The model under review builds one solid part; all positions refer to its coordinate system, in mm. A direction names the side the tool comes from. Coordinates: 2 decimals unless noted, no trailing zeros. Write each loop counter-clockwise with the first axis right and the second up, starting at its lowest first coordinate (ties: lowest second). Pieces come first, ordered by that corner, then holes.
1) Add section A-A, the plane y = 0. Give the number of separate pieces and of enclosed holes in the cut face, then the cut area to 3 significant figures.
2) For line 1 (Y direction, x = 1.25, z = -1.5); line 2 (Y direction, x = 2.75, z = 0); line 3 (Y direction, x = 4.5, z = 0), list the stretches that pass through material, from the lowest coordinate up.
3) Mouldability with a two-part tool opening along Z and no side actions: class faces 4 (the flat face through (0, 3, -3)), 5 (the conical face through (3.08, -0.63, -14.27)), 6 (the cylindrical face through (3.219, 3.514, -7.457)) as released by +Z, released by -Z, zero draft, split by the parting line, or undercut.
4) Add section B-B, the plane x = 2.75. State the section outline as (y, z) points (1 decimal), then the cut area to 3 significant figures.
5) Machinability: for faces 1 (the cylindrical face through (3.219, 0.445, 6.833)), 2 (the flat face through (6.35, 3, 3)), 3 (the conical face through (3.294, 12.703, 6.607)), which of the approach directions +Z, -Z, +X, -X, +Y, -Y give a long, thin tool a straight path to every point of the face, cutting with its end or side? Answer none if there is none.
6) For P1, Ø1.5, axis at x = 2, z = 12, coming from the -Y side; P2, Ø2, axis at x = 1, y = 10, coming from the -Z side; P3, Ø1.5, axis at x = 3, z = -9, coming from the -Y side, all flat-tipped, find the tip position at first contact; note any pin that passes through.
from build123d import *

# Parameters (mm, degrees)
CUT_EXTRUDE1_DEPTH      = 25.4561342
CUT_EXTRUDE1_DEPTH_BACK = 25.4561342


with BuildPart() as part:
    # Sketch1 → Revolve1 (revolve)
    with BuildSketch(Plane.XY, mode=Mode.PRIVATE) as revolve1_sk:
        Polygon((1.27, 16.7), (3.175, 14.16), (5.08, 16.7), (6.35, 16.7), (6.35, 4), (0, 4), (0, 16.7), align=None)
    revolve(revolve1_sk.sketch.rotate(Axis((0, 0, 0), (1, 0, 0)), 90), axis=Axis((0, 0, 0), (1, 0, 0)))

    # Sketch2 → Cut-Extrude1 (cut, two sides: drawn at the far end of the back side and taken through both)
    with BuildSketch(Plane.ZY.offset(-CUT_EXTRUDE1_DEPTH_BACK)):
        with BuildLine():
            ThreePointArc((-5.174909182, -4.484253782), (-6.96638667, -4.356158459), (-7.094481993, -6.147635947))
            ThreePointArc((-7.094481993, -6.147635947), (-4.201848282, -8.394615744), (-0.66952126, -9.363591392))
            ThreePointArc((-0.66952126, -9.363591392), (0.687821691, -8.187402584), (-0.488367117, -6.830059633))
            ThreePointArc((-0.488367117, -6.830059633), (-3.064943047, -6.123262296), (-5.174909182, -4.484253782))
        make_face()
        with BuildLine():
            ThreePointArc((-1.296023102, 6.723729704), (-0.289350555, 8.211147057), (-1.776767907, 9.217819605))
            ThreePointArc((-1.776767907, 9.217819605), (-5.169026349, 7.836215226), (-7.774347387, 5.261618115))
            ThreePointArc((-7.774347387, 5.261618115), (-7.434409475, 3.498030233), (-5.670821594, 3.837968145))
            ThreePointArc((-5.670821594, 3.837968145), (-3.77042918, 5.715949687), (-1.296023102, 6.723729704))
        make_face()
        with BuildLine():
            ThreePointArc((6.470932282, -2.239475923), (7.255737222, -3.854988599), (8.871249898, -3.070183659))
            ThreePointArc((8.871249898, -3.070183659), (9.370874629, 0.558400517), (8.443868645, 4.101973277))
            ThreePointArc((8.443868645, 4.101973277), (6.746587782, 4.68937235), (6.159188708, 2.992091487))
            ThreePointArc((6.159188708, 2.992091487), (6.835372224, 0.407312608), (6.470932282, -2.239475923))
        make_face()
    extrude(amount=CUT_EXTRUDE1_DEPTH + CUT_EXTRUDE1_DEPTH_BACK, mode=Mode.SUBTRACT)


solid = part.part
Geometry results:
1. separate pieces: 3
1. enclosed holes: 0
1. area: 135 mm2
2. line 1: y = -16.63 to -9.27, -6.68 to -3.71, 3.71 to 6.68, 9.24 to 16.63
2. line 2: y = -14.73 to -9.23, -6.97 to -4, 4 to 14.73
2. line 3: y = -15.93 to -9.23, -6.97 to -4, 4 to 15.93
3. face 4: zero draft
3. face 5: split by the parting line
3. face 6: undercut
4. outline: circle Ø29.5 at (0, 0); hole (-9.4, -0.7) arc R9.4 ccw to (-6.1, -7.1) arc R1.3 ccw to (-4.5, -5.2) arc R6.8 cw to (-6.8, -0.5) arc R1.3 ccw to start; hole circle Ø8 at (0, 0); hole (-3.1, 8.9) arc R1.3 ccw to (-2.2, 6.5) arc R6.8 cw to (3, 6.2) arc R1.3 ccw to (4.1, 8.4) arc R9.4 ccw to start; hole (3.8, -5.7) arc R1.3 ccw to (5.3, -7.8) arc R9.4 ccw to (9.2, -1.8) arc R1.3 ccw to (6.7, -1.3) arc R6.8 cw to start
4. area: 567 mm2
5. face 1: +X, -X
5. face 2: +Z, -Z, +X, +Y, -Y
5. face 3: none
6. P1: stops at y = -11.84
6. P2: stops at z = -14.07
6. P3: stops at y = -12.6
